```python
from build123d import *

# Parameters (mm, degrees)
F0_R     = 63.5
F0_R_2   = 44.45
F1_DEPTH = 6.35
F2_R     = 31.75
F2_R_2   = 12.7
F3_DEPTH = 6.35
F4_R     = 31.75
F4_R_2   = 12.7
F5_DEPTH = 6.35
F8_R     = 38.1


# Not quite as in the source:
# - two fillets or chamfers of one size are made in one step


with BuildPart() as f1:
    # F0 (on Top) → F1 (new body)
    with BuildSketch(Plane.XY):
        Circle(F0_R)
        Circle(F0_R_2, mode=Mode.SUBTRACT)
    extrude(amount=-F1_DEPTH)

    # F2 (on Top) → F3 (join)
    with BuildSketch(Plane.XY):
        with Locations((-76.2, 0)):
            Circle(F2_R)
        with Locations((-76.2, 0)):
            Circle(F2_R_2, mode=Mode.SUBTRACT)
    extrude(amount=-F3_DEPTH)

    # F4 (on Top) → F5 (join)
    with BuildSketch(Plane.XY):
        with Locations((76.2, 5.3983563557)):
            Circle(F4_R)
        with Locations((76.2, 5.3983563557)):
            Circle(F4_R_2, mode=Mode.SUBTRACT)
    extrude(amount=-F5_DEPTH)

    # F6: union 

    # F7: union 

    # F8
    f8_edges = [f1.edges().sort_by_distance(p)[0] for p in [
        (-57.94375, 25.976371, -3.175),
        (56.016218, 29.907078, -3.175),
        (59.673087, -21.711119, -3.175),
        (-57.94375, -25.976371, -3.175),
    ]]
    fillet(f8_edges, radius=F8_R)


solid = f1.part
```
Geometry: final body of the model. Coordinates: model frame, mm. Coordinates: 2 decimals unless noted, no trailing zeros. Order: outer loops, then holes, each group sorted by start corner. A loop starts at its lowest first (then second) coordinate and runs counter-clockwise, first axis right, second up. Notation, with made-up numbers: M 75,-37.5 L 84,-37.5 A16 cw 84,-11.5 Z; hole C 83.25,12.25 d10. An arc over 180 degrees is marked long. Answer as CSV lines item,"result".
Q1. First-contact query: P1, Ø23, axis at x = 76.2, y = 5.4, coming from the -Z side; P2, Ø3, axis at y = -17.5, z = -5, coming from the -X side; P3, Ø3, axis at x = 85.5, z = -1, coming from the +Y side; P4, Ø1, axis at y = 17.5, z = -3, coming from the -X side. Flat tips, straight axial feed; report the tip coordinate or a pass-through.
Answers:
P1,"passes through"
P2,"stops at x = -103.62"
P3,"stops at y = 36.18"
P4,"stops at x = -103.02"
Q2. Section C-C on y = 24.5. Return the cut outline in (x, z).
Answers:
outline,"M -96.39,-6.35 L -37.09,-6.35 L -37.09,0 L -96.39,0 Z; M 37.09,-6.35 L 101.56,-6.35 L 101.56,0 L 37.09,0 Z"
Q3. Draft query along Y for faces 1 (the cylindrical face through (107.913, 6.929, -3.131)), 2 (the flat face through (46, 1, 0)), 3 (the cylindrical face through (-64.086, 3.815, -3.131)). Return one class per face: pulls with the +Y half, pulls with the -Y half, needs draft (parallel to the pull), parting line crosses it, or undercut.
Answers:
face 1,"parting line crosses it"
face 2,"needs draft"
face 3,"undercut"
Q4. Section B-B on y = 0. Return the cut outline in (x, z).
Answers:
outline,"M -107.95,-6.35 L -88.9,-6.35 L -88.9,0 L -107.95,0 Z; M -63.5,-6.35 L -44.45,-6.35 L -44.45,0 L -63.5,0 Z; M 44.45,-6.35 L 64.7,-6.35 L 64.7,0 L 44.45,0 Z; M 87.7,-6.35 L 107.49,-6.35 L 107.49,0 L 87.7,0 Z"
Q5. Section D-D on z = -3. Count the separate pieces of the cut face and the enclosed holes in it, and give its area (3 significant figures).
Answers:
separate pieces,"1"
enclosed holes,"3"
area,"10,800 mm^2"
Q6. Line query: probe 1 along Y at (x, z) = (0, -2.75); probe 2 along X at (y, z) = (5, -5.5); probe 3 along Y at (x, z) = (-76.2, -2). Output: solid intervals per line, ascending. Write a range as [from, to].
Answers:
probe 1,"y = [-63.5, -44.45], [44.45, 63.5]"
probe 2,"x = [-107.55, -87.87], [-64.53, -44.17], [44.17, 63.51], [88.89, 107.95]"
probe 3,"y = [-31.75, -12.7], [12.7, 31.75]"
Q7. Section A-A on x = 0. Return the cut outline in (y, z).
Answers:
outline,"M -63.5,-6.35 L -44.45,-6.35 L -44.45,0 L -63.5,0 Z; M 44.45,-6.35 L 63.5,-6.35 L 63.5,0 L 44.45,0 Z"
